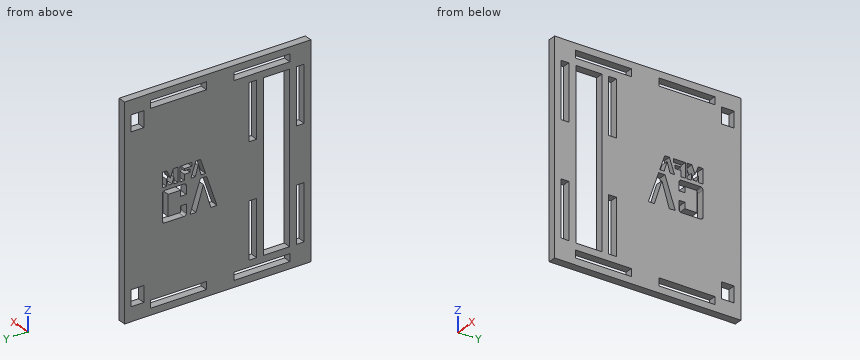
```python
from build123d import *

# Parameters (mm, degrees)
F0_W     = 140
F0_H     = 157.3
F0_W_2   = 5.7
F0_H_2   = 42
F0_W_3   = 42
F0_H_3   = 5.7
F0_W_4   = 9.525
F0_H_4   = 12
F0_W_5   = 19.719037
F0_H_5   = 125.9
F1_DEPTH = 5.8


with BuildPart() as f1:
    # F0 (on Right) → F1 (new body)
    with BuildSketch(Plane.YZ):
        Rectangle(F0_W, F0_H)
        with Locations((-62.15, -41.95)):
            Rectangle(F0_W_2, F0_H_2, mode=Mode.SUBTRACT)
        with Locations((-33.3, -70.8)):
            Rectangle(F0_W_3, F0_H_3, mode=Mode.SUBTRACT)
        with Locations((-26.45, -41.95)):
            Rectangle(F0_W_2, F0_H_2, mode=Mode.SUBTRACT)
        with Locations((29.475, -70.8)):
            Rectangle(F0_W_3, F0_H_3, mode=Mode.SUBTRACT)
        with Locations((60.2375, -61.95)):
            Rectangle(F0_W_4, F0_H_4, mode=Mode.SUBTRACT)
        Polygon((5.084475, -16.499415), (0.537139, -16.43919), (8.306721, 6.508208), (13.00455, 6.508208), (20.774202, -16.43919), (16.257049, -16.499415), (10.685818, 1.479072), align=None, mode=Mode.SUBTRACT)
        with BuildLine():
            Line((25.34413, 6.508206), (39.782841, 6.508207))
            ThreePointArc((39.782841, 6.508207), (41.055633, 5.981), (41.582841, 4.708207))
            Line((41.582841, 4.708207), (41.582841, -14.699417))
            ThreePointArc((41.582841, -14.699417), (41.055633, -15.972209), (39.782841, -16.499417))
            Line((39.782841, -16.499417), (25.34413, -16.499416))
            ThreePointArc((25.34413, -16.499416), (24.071338, -15.972208), (23.54413, -14.699416))
            Line((23.54413, -14.699416), (23.54413, -8.248033))
            Line((23.54413, -8.248033), (27.971016, -8.248033))
            Line((27.971016, -8.248033), (27.971016, -12.855594))
            Line((27.971016, -12.855594), (37.155955, -12.855594))
            Line((37.155955, -12.855594), (37.155955, 2.864386))
            Line((37.155955, 2.864386), (27.971016, 2.864386))
            Line((27.971016, 2.864386), (27.971016, -1.472232))
            Line((27.971016, -1.472232), (23.54413, -1.472232))
            Line((23.54413, -1.472232), (23.54413, 4.708206))
            ThreePointArc((23.54413, 4.708206), (24.071338, 5.980998), (25.34413, 6.508206))
        make_face(mode=Mode.SUBTRACT)
        with Locations((-44.159518, 0)):
            Rectangle(F0_W_5, F0_H_5, mode=Mode.SUBTRACT)
        with Locations((-62.15, 41.95)):
            Rectangle(F0_W_2, F0_H_2, mode=Mode.SUBTRACT)
        with Locations((-26.45, 41.95)):
            Rectangle(F0_W_2, F0_H_2, mode=Mode.SUBTRACT)
        with Locations((-33.3, 70.8)):
            Rectangle(F0_W_3, F0_H_3, mode=Mode.SUBTRACT)
        Polygon((16.363741, 19.928689), (20.179323, 8.915522), (16.855157, 8.886603), (14.62936, 16.402229), (12.418023, 8.886603), (9.064938, 8.915522), (12.88059, 19.928689), align=None, mode=Mode.SUBTRACT)
        Polygon((20.655928, 13.251439), (20.655928, 15.766287), (25.020764, 15.766287), (25.020764, 17.269385), (19.384044, 17.269385), (19.384044, 19.928689), (28.287162, 19.928689), (28.287162, 8.886603), (25.020764, 8.886603), (25.020764, 13.251439), align=None, mode=Mode.SUBTRACT)
        Polygon((38.345925, 13.815083), (36.944045, 9.363489), (34.313589, 9.363489), (32.911639, 13.815083), (32.911639, 8.886603), (29.746389, 8.886603), (29.746389, 19.928689), (33.186231, 19.928689), (35.599863, 14.002917), (38.085792, 19.928689), (41.554554, 19.928689), (41.554554, 8.886603), (38.345925, 8.886603), align=None, mode=Mode.SUBTRACT)
        with Locations((29.475, 70.8)):
            Rectangle(F0_W_3, F0_H_3, mode=Mode.SUBTRACT)
        with Locations((60.2375, 61.95)):
            Rectangle(F0_W_4, F0_H_4, mode=Mode.SUBTRACT)
    extrude(amount=F1_DEPTH)


solid = f1.part
```
Check sheet for the modelled part. Datum: model origin and axes. Units: mm. Round coordinates to 2 decimals unless told otherwise and drop trailing zeros. Loops run counter-clockwise (first coordinate to the right, second up) from the corner with the lowest first, then second, coordinate; pieces in that order, holes last. Notation, with made-up numbers: M 40,51 L 51,51 A6 cw 51,57 Z; hole C 88,14.5 d10. An arc over 180 degrees is marked long. Answer as a JSON object with one key per item and string values.
1. Section check C-C (x = 1.35). State how many separate pieces and enclosed holes the cut face has, plus the area to 3 significant figures.
Reply:
{"separate pieces": "1", "enclosed holes": "16", "area": "16,700 mm²"}
2. Section check B-B (z = -65.5). Record the boundary of the cut face in (x, y) (3 decimals), plus the area to 3 significant figures.
Reply:
{"outline": "M 0,-70 L 5.8,-70 L 5.8,55.475 L 0,55.475 Z; M 0,65 L 5.8,65 L 5.8,70 L 0,70 Z", "area": "757 mm²"}
3. Scan lines: line 1 (Y direction, x = 3.15, z = 51); line 2 (Z direction, x = 2, y = -49); line 3 (Y direction, x = 4.5, z = -70) (3 decimals). Record each from-to range of solid material in increasing order.
Reply:
{"line 1": "y = -70 to -65, -59.3 to -54.02, -34.3 to -29.3, -23.6 to 70", "line 2": "z = -78.65 to -73.65, -67.95 to -62.95, 62.95 to 67.95, 73.65 to 78.65", "line 3": "y = -70 to -54.3, -12.3 to 8.475, 50.475 to 70"}
4. Section check A-A (z = -43.5). Record the boundary of the cut face in (x, y), plus the area to 3 significant figures.
Reply:
{"outline": "M 0,-70 L 5.8,-70 L 5.8,-65 L 0,-65 Z; M 0,-59.3 L 5.8,-59.3 L 5.8,-54.02 L 0,-54.02 Z; M 0,-34.3 L 5.8,-34.3 L 5.8,-29.3 L 0,-29.3 Z; M 0,-23.6 L 5.8,-23.6 L 5.8,70 L 0,70 Z", "area": "632 mm²"}
